Can you work these out from the model? Positions are in its coordinate system, mm. A direction names the side the tool comes from. Coordinates: 2 decimals unless noted, no trailing zeros. Put each result on its own line as item: value. Start each with the question number.
from build123d import *

# Parameters (mm, degrees)
F0_W     = 40
F0_H     = 30
F1_DEPTH = 110
F1_TAPER = -3
F2_W     = 35
F2_H     = 25
F3_DEPTH = 10


with BuildPart() as f1:
    # F0 (on Top) → F1 (new body)
    with BuildSketch(Plane.XY):
        with Locations((-30.053210146, -58.0066898444)):
            Rectangle(F0_W, F0_H)
    extrude(amount=F1_DEPTH, taper=F1_TAPER)

    # F2 (on face) → F3 (cut)
    with BuildSketch(Plane(origin=(0, 0, 0), x_dir=(1, 0, 0), z_dir=(0, 0, -1))):
        with Locations((-30.053210146, 58.0066898444)):
            Rectangle(F2_W, F2_H)
    extrude(amount=-F3_DEPTH, mode=Mode.SUBTRACT)


solid = f1.part
Q1. On a 3-axis mill with a long thin cutter (end or side, diameter ignored), from which of +Z, -Z, +X, -X, +Y, -Y can I reach the whole of each face in a straight line? I mean faces 1 (the flat face through (-31, -58, 110)), 2 (the flat face through (-47.553, -58, 5)). Say none if no direction works.
Q2. Please list where these lines run through material, in increasing order: line 1 along Z through (x, y) = (-21, -64); line 2 along Y through (x, z) = (-20, 27.5); line 3 along Y through (x, z) = (-30, 64). Write a range as [from, to].
Q3. We'd pull the mould along Y, two halves only. Please class faces 3 (the flat face through (-32, -71, 0)), 4 (the flat face through (-30, -58, 10)): released by +Y, released by -Y, zero draft, split by the parting line, or undercut.
Q4. Will these pins go through, and if not, where does the flat tip stop? pin 1 (6 mm diameter, centred on y = -45.5, z = 68, fed in from -X); pin 2 (1.5 mm diameter, centred on x = -36, z = 96, fed in from -Y); pin 3 (11 mm diameter, centred on y = -59.5, z = 7, fed in from +X).
Calculated:
1. face 1: +Z, +X, -X, +Y, -Y
1. face 2: -Z
2. line 1: [10, 110]
2. line 2: [-74.45, -41.57]
2. line 3: [-76.36, -39.65]
3. face 3: zero draft
3. face 4: undercut
4. pin 1: x = -53.77
4. pin 2: y = -78.08
4. pin 3: x = -9.4
